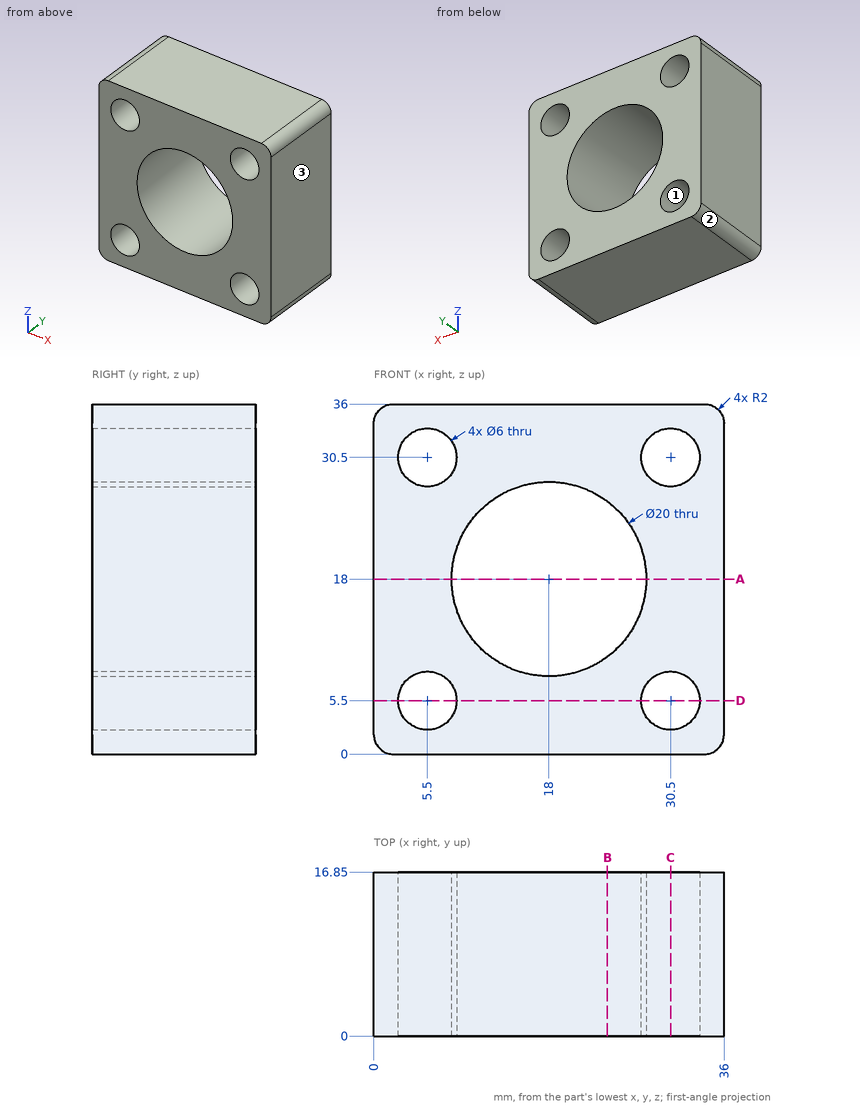
Answer from the drawing. Dimensions are ordinates in mm from the lowest x, y and z of the part. Give positions to 0.01 mm unless a question says otherwise; leave off trailing zeros. Loops run counter-clockwise (first coordinate to the right, second up) from the corner with the lowest first, then second, coordinate; pieces in that order, holes last. Notation, with made-up numbers: (-17.5, 56) - (-3.5, 56) arc R12 cw to (-3.5, 67) - close; hole circle Ø1 at (19.25, 72.5). An arc over 180 degrees is marked (long way). Answer as CSV lines item,"result". Start each with the question number.
Item 1: A cutting plane is placed at A-A on z = 18. Determine the outline of the cut face in (x, y), then the cut area to 3 significant figures.
Item 2: Find the intervals of material crossed by line 1 (X direction, y = 13.5, z = 30.5); line 2 (Z direction, x = 29, y = 9.5), in increasing order. Write a range as from..to.
Item 3: The mould has two halves that part along X. Classify the marked faces 1, 2 and 3: +X half, -X half, draft (parallel to the pull), parting line (faces both ways), or undercut.
Item 4: A cutting plane is placed at C-C on x = 30.5. Determine the outline of the cut face in (y, z).
Item 5: A cutting plane is placed at D-D on z = 5.5. Determine the outline of the cut face in (x, y).
Item 6: A cutting plane is placed at B-B on x = 24. Determine the outline of the cut face in (y, z), then the cut area to 3 significant figures.
Item 7: This flat-tipped pin is pushed along its axis until it touches: pin 1 (7 mm diameter, centred on x = 30.5, z = 5.5, fed in from +Y). Where does it stop, or does it pass through?
Found:
1,outline,"(0, 0) - (8, 0) - (8, 16.85) - (0, 16.85) - close; (28, 0) - (36, 0) - (36, 16.85) - (28, 16.85) - close"
1,area,"270 mm^2"
2,line 1,"x = 0..2.5, 8.5..27.5, 33.5..36"
2,line 2,"z = 0..2.9, 8.1..27.9, 33.1..36"
3,face 1,"undercut"
3,face 2,"-X half"
3,face 3,"+X half"
4,outline,"(0, 0) - (16.85, 0) - (16.85, 2.5) - (0, 2.5) - close; (0, 8.5) - (16.85, 8.5) - (16.85, 27.5) - (0, 27.5) - close; (0, 33.5) - (16.85, 33.5) - (16.85, 36) - (0, 36) - close"
5,outline,"(0, 0) - (2.5, 0) - (2.5, 16.85) - (0, 16.85) - close; (8.5, 0) - (27.5, 0) - (27.5, 16.85) - (8.5, 16.85) - close; (33.5, 0) - (36, 0) - (36, 16.85) - (33.5, 16.85) - close"
6,outline,"(0, 0) - (16.85, 0) - (16.85, 10) - (0, 10) - close; (0, 26) - (16.85, 26) - (16.85, 36) - (0, 36) - close"
6,area,"337 mm^2"
7,pin 1,"stops at y = 16.85"
